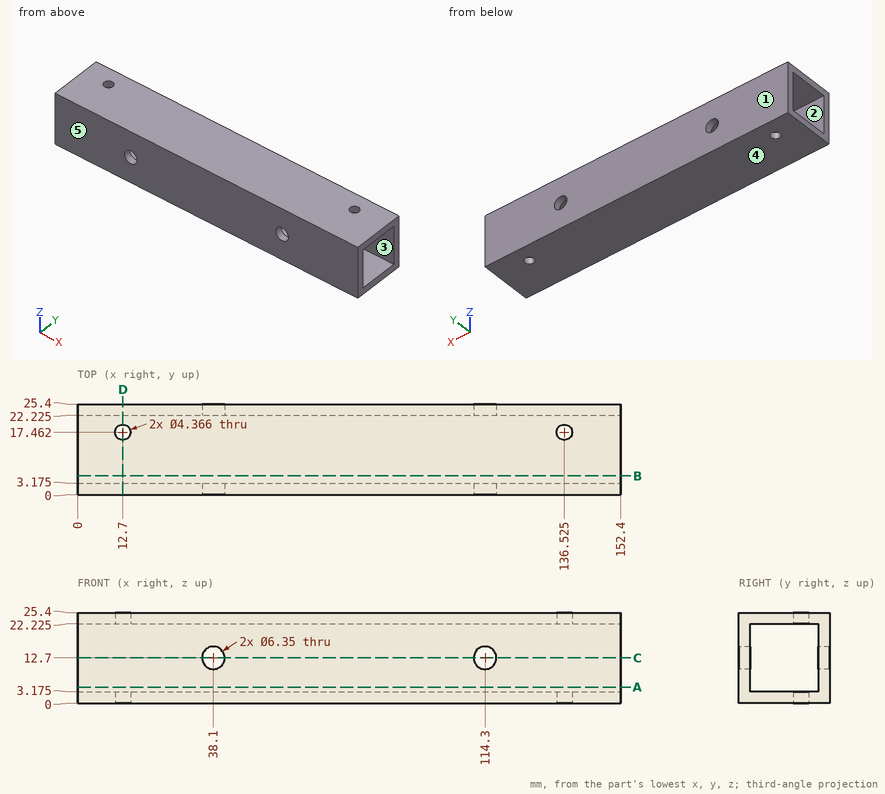
Input: dimensioned drawing with shaded views. Units: mm. Origin: part minimum x, y, z. A direction names the side the tool comes from. Give positions to 0.01 mm unless a question says otherwise; leave off trailing zeros. Loops run counter-clockwise (first coordinate to the right, second up) from the corner with the lowest first, then second, coordinate; pieces in that order, holes last. Notation, with made-up numbers: (-3.5, -25) -> (42.5, -25) arc R24 ccw to (42.5, -2) -> close; hole circle Ø3 at (-26, 88). An arc over 180 degrees is marked (long way). Return JSON: item names as keys, results as strings.
Item 1: Mould query, pull axis Z, two halves, no side actions, for the marked faces 3, 4 and 5. Classes: released by +Z, released by -Z, zero draft, split by the parting line, or undercut.
Filled in:
{"face 3": "undercut", "face 4": "released by -Z", "face 5": "zero draft"}
Item 2: Pin query (flat end, axial travel): P1, Ø4, axis at x = 136.52, y = 17.46, coming from the +Z side. Return the tip coordinate at first contact, or that it passes through.
Filled in:
{"P1": "through"}
Item 3: Section D-D, the plane x = 12.7. Output: boundary loops of the cut face in (y, z) (1 decimal).
Filled in:
{"outline": "(0, 0) -> (15.3, 0) -> (15.3, 3.2) -> (3.2, 3.2) -> (3.2, 22.2) -> (15.3, 22.2) -> (15.3, 25.4) -> (0, 25.4) -> close; (19.6, 0) -> (25.4, 0) -> (25.4, 25.4) -> (19.6, 25.4) -> (19.6, 22.2) -> (22.2, 22.2) -> (22.2, 3.2) -> (19.6, 3.2) -> close"}
Item 4: Section C-C, the plane z = 12.7. Output: boundary loops of the cut face in (x, y) (1 decimal).
Filled in:
{"outline": "(0, 0) -> (34.9, 0) -> (34.9, 3.2) -> (0, 3.2) -> close; (0, 22.2) -> (34.9, 22.2) -> (34.9, 25.4) -> (0, 25.4) -> close; (41.3, 0) -> (111.1, 0) -> (111.1, 3.2) -> (41.3, 3.2) -> close; (41.3, 22.2) -> (111.1, 22.2) -> (111.1, 25.4) -> (41.3, 25.4) -> close; (117.5, 0) -> (152.4, 0) -> (152.4, 3.2) -> (117.5, 3.2) -> close; (117.5, 22.2) -> (152.4, 22.2) -> (152.4, 25.4) -> (117.5, 25.4) -> close"}
Item 5: Access query for the marked faces 1 and 2. Directions: +Z, -Z, +X, -X, +Y, -Y. A direction counts if a zero-diameter tool reaches every point of the face in a straight line with its end or side. Return the directions, or none.
Filled in:
{"face 1": "+Z, -Z, +X, -X, +Y", "face 2": "+X, -X"}
Item 6: Line query: line 1 (X direction, y = 0.8, z = 12.7) (1 decimal); line 2 (Y direction, x = 53.5, z = 10.25) (1 decimal). Output: solid intervals per line, ascending.
Filled in:
{"line 1": "0 to 34.9, 41.3 to 111.1, 117.5 to 152.4", "line 2": "0 to 3.2, 22.2 to 25.4"}
Item 7: Section A-A, the plane z = 4.5. Output: boundary loops of the cut face in (x, y) (1 decimal).
Filled in:
{"outline": "(0, 0) -> (152.4, 0) -> (152.4, 3.2) -> (0, 3.2) -> close; (0, 22.2) -> (152.4, 22.2) -> (152.4, 25.4) -> (0, 25.4) -> close"}
